Verification items for the finished model (mm, model axes). A direction names the side the tool comes from. Round coordinates to 2 decimals unless told otherwise and drop trailing zeros. Write each loop counter-clockwise with the first axis right and the second up, starting at its lowest first coordinate (ties: lowest second). Pieces come first, ordered by that corner, then holes. Notation, with made-up numbers: M 37,17.5 L 72,17.5 A20 ccw 72,24.5 Z; hole C 48,80 d6. An arc over 180 degrees is marked long. One line per item, written item: value. Start each with the question number.
Item 1: Tool access check on faces 5 (the face through (-0.48, 4.75, 20.12)), 6 (the face through (-0.2, 6.7, -12.8)), 7 (the face through (-34.75, 1.6, 12.36)). Record the directions out of +Z, -Z, +X, -X, +Y, -Y that give a thin tool (end or side, any length) a straight path to the whole face; none if there is none.
Item 2: Section check C-C, the plane x = -11. Record the cut outline in (y, z), then the cut area to 3 significant figures.
Item 3: Section check B-B, the plane z = -20. Record the cut outline in (x, y) (3 decimals).
Item 4: Draft check along Z on faces 1 (the face through (0.705, 1.604, 14.285)), 2 (the face through (-63.5, 5, 0)), 3 (the face through (-1, 5, -30)), 4 (the face through (-34.37, 4.6, 19.9)). Enter one of: +Z half, -Z half, draft (parallel to the pull), parting line (faces both ways), or undercut.
Item 5: Section check A-A, the plane x = -31.75. Record the cut outline in (y, z), then the cut area to 3 significant figures.
Item 6: Section check D-D, the plane y = 8.25. State how many separate pieces and enclosed holes the cut face has, then the cut area to 3 significant figures.
Item 7: Gauge pin test, flat end, axial feed: pin 1 (4.5 mm diameter, centred on x = -31.75, z = 11.11, fed in from -Y). Record the tip position at first contact, or that the pin passes through.
Item 8: Thickness scan on probe 1 along X at (y, z) = (3.5, -23.5); probe 2 along X at (y, z) = (9.5, -15); probe 3 along Z at (x, y) = (-36.5, 7.5). Record the ranges inside material, lowest first. Write a range as from..to.
from build123d import *

# Parameters (mm, degrees)
SKETCH1_W                      = 127
SKETCH1_H                      = 60
BOSS_EXTRUDE1_DEPTH            = 10
CUT_EXTRUDE1_START             = -5.08
SKETCH3_R                      = 7.525
CUT_EXTRUDE1_DEPTH             = 24.05
CUT_EXTRUDE2_REACH             = 127.954
SKETCH4_R                      = 4.25
CUT_EXTRUDE2_DIRECTION_2_REACH = 127.954
CUT_EXTRUDE3_START             = -68.74
SKETCH5_R                      = 5.25
SKETCH5_R_2                    = 4.25
CUT_EXTRUDE3_DEPTH             = 68.74
CBORE_FOR_M3_SHCS1_D           = 3.4
CBORE_FOR_M3_SHCS1_CBORE_D     = 6.5
CBORE_FOR_M3_SHCS1_CBORE_DEPTH = 3.254


with BuildPart() as part:
    # Sketch1 → Boss-Extrude1 (new body)
    with BuildSketch(Plane(origin=(0, 0, 0), x_dir=(1, 0, 0), z_dir=(0, 1, 0))):
        Rectangle(SKETCH1_W, SKETCH1_H)
    extrude(amount=BOSS_EXTRUDE1_DEPTH)

    # Sketch3 → Cut-Extrude1 (cut)
    with BuildSketch(Plane.ZY.offset(63.5).offset(CUT_EXTRUDE1_START)):
        with Locations((-20, 10)):
            Circle(SKETCH3_R)
        with Locations((20, 10)):
            Circle(SKETCH3_R)
    cut_extrude1 = extrude(amount=-CUT_EXTRUDE1_DEPTH, mode=Mode.SUBTRACT)

    # Mirror1: Cut-Extrude1 across plane
    add(cut_extrude1.mirror(Plane(origin=(0, 0, 0), x_dir=(0, 0, 1), z_dir=(1, 0, 0))), mode=Mode.SUBTRACT)

    # Sketch4 → Cut-Extrude2 (cut, up to next)
    with BuildSketch(Plane(origin=(-58.42, 0, 0), x_dir=(0, 0, -1), z_dir=(1, 0, 0)), mode=Mode.PRIVATE) as cut_extrude2_sk1:
        with Locations((20, 10)):
            Circle(SKETCH4_R)
    cut_extrude2_tool1 = extrude(cut_extrude2_sk1.sketch, amount=-CUT_EXTRUDE2_REACH, mode=Mode.PRIVATE) & part.part
    cut_extrude2 = cut_extrude2_tool1.solids().sort_by_distance((-58.42, 10, -20))[0]
    add(cut_extrude2, mode=Mode.SUBTRACT)

    # Cut-Extrude2 direction 2: up to this face of the body (flat: up to its plane)
    cut_extrude2_direction_2_end = Plane(part.part.faces().sort_by_distance((63.5, 5, 0))[0])
    # Sketch4 → Cut-Extrude2 direction 2 (cut, up to the picked face)
    with BuildSketch(Plane(origin=(-58.42, 0, 0), x_dir=(0, 0, -1), z_dir=(1, 0, 0)), mode=Mode.PRIVATE) as cut_extrude2_direction_2_sk1:
        with Locations((20, 10)):
            Circle(SKETCH4_R)
    cut_extrude2_direction_2_tool1 = split(extrude(cut_extrude2_direction_2_sk1.sketch, amount=CUT_EXTRUDE2_DIRECTION_2_REACH, mode=Mode.PRIVATE), bisect_by=cut_extrude2_direction_2_end, keep=Keep.BOTH, mode=Mode.PRIVATE)
    cut_extrude2_direction_2 = cut_extrude2_direction_2_tool1.solids().sort_by(Axis((-58.42, 10, -20), (1, 0, 0)))[0]
    add(cut_extrude2_direction_2, mode=Mode.SUBTRACT)

    # Mirror2: Cut-Extrude2, Cut-Extrude2 direction 2 across plane
    add(cut_extrude2.mirror(Plane.XY), mode=Mode.SUBTRACT)
    add(cut_extrude2_direction_2.mirror(Plane.XY), mode=Mode.SUBTRACT)

    # Sketch5 → Cut-Extrude3 (cut)
    with BuildSketch(Plane(origin=(34.37, 0, 0), x_dir=(0, 0, -1), z_dir=(1, 0, 0)).offset(CUT_EXTRUDE3_START)):
        with Locations((-20, 10)):
            Circle(SKETCH5_R)
        with Locations((-20, 10)):
            Circle(SKETCH5_R_2, mode=Mode.SUBTRACT)
    cut_extrude3 = extrude(amount=CUT_EXTRUDE3_DEPTH, mode=Mode.SUBTRACT)

    # Mirror3: Cut-Extrude3 across plane
    add(cut_extrude3.mirror(Plane.XY), mode=Mode.SUBTRACT)

    # CBORE for M3 SHCS1 (through all)
    with Locations(Plane(origin=(0, 0, 0), x_dir=(-1, 0, 0), z_dir=(0, -1, 0))):
        with Locations((-31.75, -11.1125), (0, -11.1125), (31.75, -11.1125), (-31.75, 11.1125), (0, 11.1125), (31.75, 11.1125)):
            CounterBoreHole(CBORE_FOR_M3_SHCS1_D / 2, CBORE_FOR_M3_SHCS1_CBORE_D / 2, CBORE_FOR_M3_SHCS1_CBORE_DEPTH)


solid = part.part
Response values:
1. face 5: +Y
1. face 6: +Y, -Y
1. face 7: -Y
2. outline: M 0,-30 L 10,-30 L 10,-25.25 A5.25 cw 10,-14.75 L 10,14.75 A5.25 cw 10,25.25 L 10,30 L 0,30 Z
2. area: 513 mm2
3. outline: M -63.5,0 L 63.5,0 L 63.5,5.75 L 58.42,5.75 L 58.42,2.475 L 34.37,2.475 L 34.37,4.75 L -34.37,4.75 L -34.37,2.475 L -58.42,2.475 L -58.42,5.75 L -63.5,5.75 Z
4. face 1: undercut
4. face 2: draft
4. face 3: -Z half
4. face 4: undercut
5. outline: M 0,-30 L 10,-30 L 10,-25.25 A5.25 cw 10,-14.75 L 10,-12.81 L 3.25,-12.81 L 3.25,-14.36 L 0,-14.36 Z; M 0,-7.86 L 3.25,-7.86 L 3.25,-9.41 L 10,-9.41 L 10,9.41 L 3.25,9.41 L 3.25,7.86 L 0,7.86 Z; M 0,14.36 L 3.25,14.36 L 3.25,12.81 L 10,12.81 L 10,14.75 A5.25 cw 10,25.25 L 10,30 L 0,30 Z
5. area: 425 mm2
6. separate pieces: 3
6. enclosed holes: 6
6. area: 4,640 mm2
7. pin 1: stops at y = 3.25
8. probe 1: x = -63.5..-58.42, -34.37..34.37, 58.42..63.5
8. probe 2: x = -63.5..-58.42, 58.42..63.5
8. probe 3: z = -30..-27.1, -12.9..12.9, 27.1..30
